Check sheet for the drawn part. Datum: minimum x, y, z corner. Units: mm. A direction names the side the tool comes from. Coordinates: 2 decimals unless noted, no trailing zeros. Write each loop counter-clockwise with the first axis right and the second up, starting at its lowest first coordinate (ties: lowest second). Pieces come first, ordered by that corner, then holes. Notation, with made-up numbers: (-23.75, 20) -> (25.25, 20) arc R18 ccw to (25.25, 51) -> close; hole circle Ø4 at (25, -3). An arc over 180 degrees is marked (long way). Answer in a Markdown table with one row per item. Add a question column.
Q1. Gauge pin test, flat end, axial feed: P1, Ø4, axis at x = 28, y = 14, coming from the -Z side. Record the tip position at first contact, or that the pin passes through.
Q2. Section check A-A, the plane z = 1. Record the boundary of the cut face in (x, y).
Q3. Release check for a two-part mould opening along Y. For the marked faces 3, 4, 5 and 6 record: pulls with the +Y half, pulls with the -Y half, needs draft (parallel to the pull), parting line crosses it, or undercut.
Q4. Section check B-B, the plane y = 23.5. Record the boundary of the cut face in (x, z), and give its area (3 significant figures).
Q5. Section check D-D, the plane y = 3. Record the boundary of the cut face in (x, z), and give its area (3 significant figures).
Q6. Tool access check on the marked faces 1 and 2. Record the directions out of +Z, -Z, +X, -X, +Y, -Y that give a thin tool (end or side, any length) a straight path to the whole face; none if there is none.
Q7. Thickness scan on line 1 (X direction, y = 13.5, z = 1.5); line 2 (X direction, y = 10, z = 4). Record the ranges inside material, lowest first.
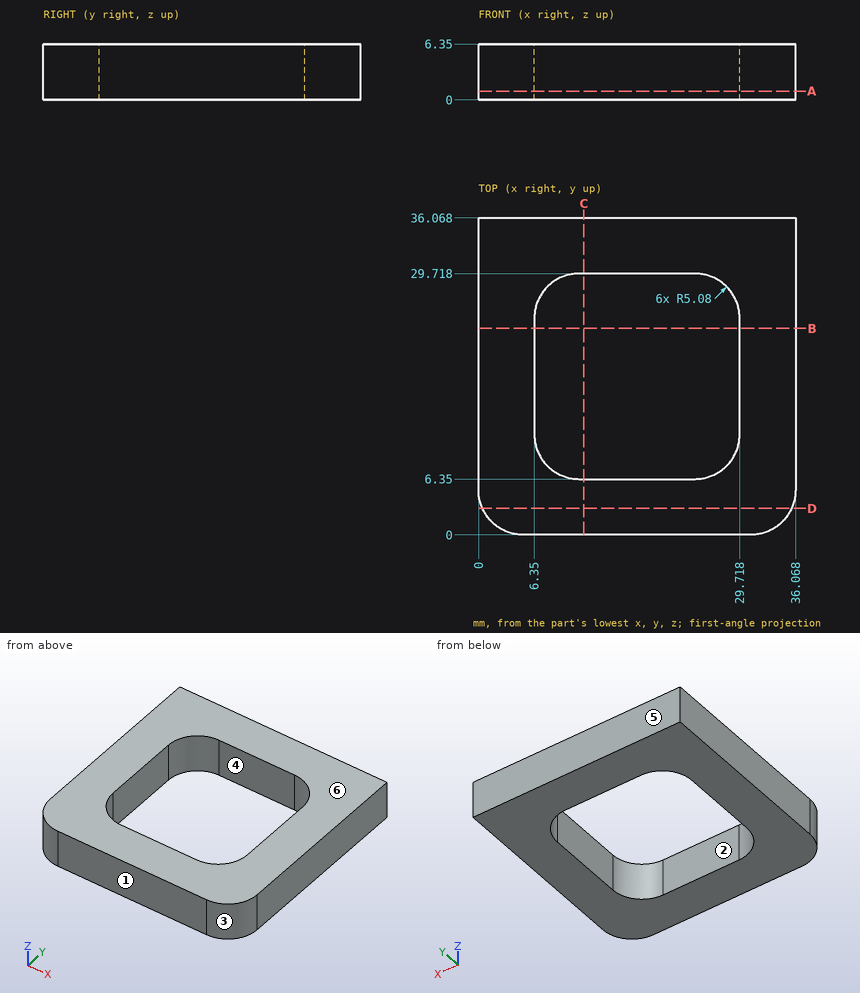
Calculated:
| question | item | result |
|---|---|---|
| 1 | P1 | stops at z = 0 |
| 2 | outline | (0, 5.08) arc R5.08 ccw to (5.08, 0) -> (30.99, 0) arc R5.08 ccw to (36.07, 5.08) -> (36.07, 36.07) -> (0, 36.07) -> close; hole (6.35, 11.43) arc R5.08 ccw to (11.43, 6.35) -> (24.64, 6.35) arc R5.08 ccw to (29.72, 11.43) -> (29.72, 24.64) arc R5.08 ccw to (24.64, 29.72) -> (11.43, 29.72) arc R5.08 ccw to (6.35, 24.64) -> close |
| 3 | face 3 | pulls with the -Y half |
| 3 | face 4 | undercut |
| 3 | face 5 | pulls with the +Y half |
| 3 | face 6 | needs draft |
| 4 | outline | (0, 0) -> (6.35, 0) -> (6.35, 6.35) -> (0, 6.35) -> close; (29.72, 0) -> (36.07, 0) -> (36.07, 6.35) -> (29.72, 6.35) -> close |
| 4 | area | 80.6 mm² |
| 5 | outline | (0.45, 0) -> (35.62, 0) -> (35.62, 6.35) -> (0.45, 6.35) -> close |
| 5 | area | 223 mm² |
| 6 | face 1 | +Z, -Z, +X, -X, -Y |
| 6 | face 2 | +Z, -Z |
| 7 | line 1 | x = 0 to 6.35, 29.72 to 36.07 |
| 7 | line 2 | x = 0 to 6.56, 29.51 to 36.07 |
